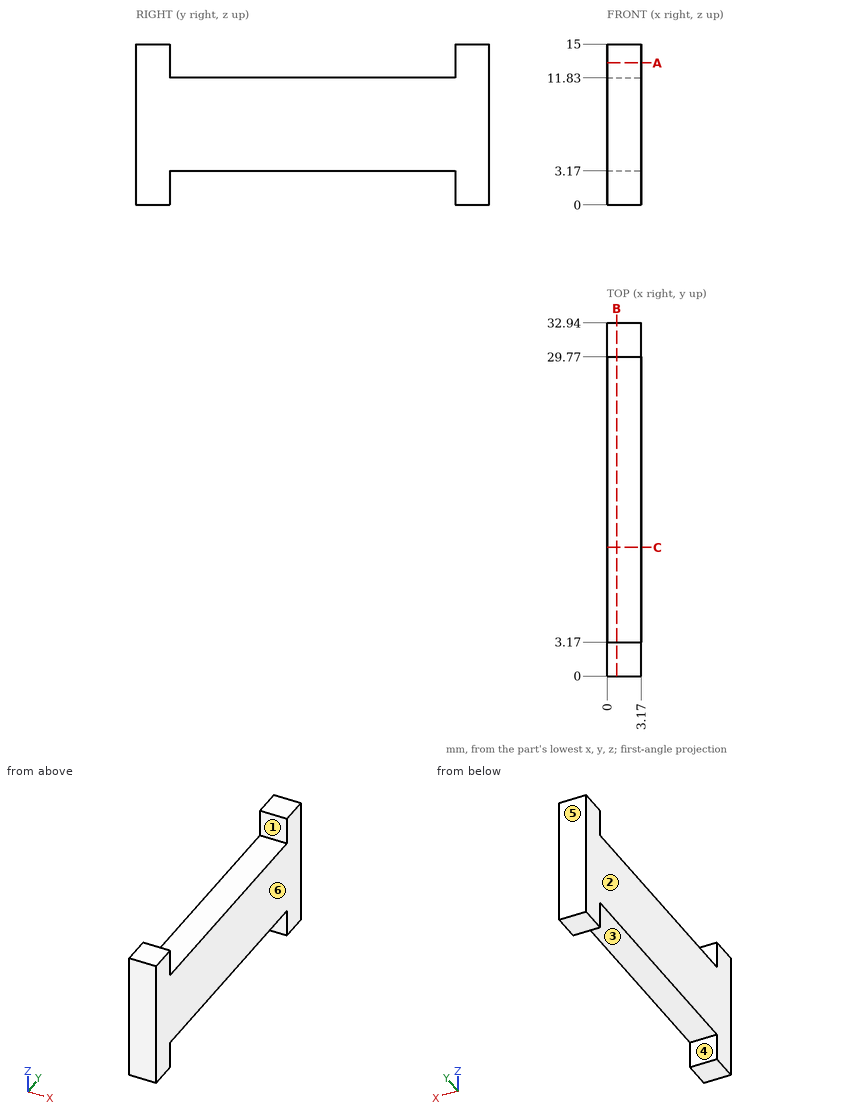
Geometry check sheet. Reference: drawing and pictorial views, mm from the part's lowest x, y, z. A direction names the side the tool comes from. Give positions to 0.01 mm unless a question says otherwise; leave off trailing zeros. Order: outer loops, then holes, each group sorted by start corner. A loop starts at its lowest first (then second) coordinate and runs counter-clockwise, first axis right, second up. Notation, with made-up numbers: M 3,-14 L 48,-14 A27 cw 48,7 Z; hole C 56,56 d9. An arc over 180 degrees is marked long. Return JSON: item names as keys, results as strings. Group by question number.
1) Mould release check, pull along Y, two halves, no side actions. Record for the marked faces 3, 4, 5 and 6: pulls with the +Y half, pulls with the -Y half, needs draft (parallel to the pull), parting line crosses it, or undercut.
2) Section check C-C on y = 12. Record the cut outline in (x, z).
3) Go/stop test with flat-tipped pins: pin 1 Ø1.6 at (x, y) = (1, 17.5) entering from -Z; pin 2 Ø1 at (x, y) = (2.5, 19.5) entering from +Z. Record where each tip stops, or that it passes through.
4) Section check A-A on z = 13.25. Record the cut outline in (x, y).
5) Section check B-B on x = 0.9. Record the cut outline in (y, z).
6) Scan lines: line 1 (Y direction, x = 1.3, z = 14.75); line 2 (Z direction, x = 1.9, y = 4). Record each from-to range of solid material in increasing order.
7) Access from +Z, -Z, +X, -X, +Y, -Y to the whole of each face (thin tool, end or side, straight path). Record for the marked faces 1 and 2.
Answer block:
{
 "1": {"face 3": "undercut", "face 4": "undercut", "face 5": "pulls with the +Y half", "face 6": "needs draft"},
 "2": {"outline": "M 0,3.17 L 3.17,3.17 L 3.17,11.83 L 0,11.83 Z"},
 "3": {"pin 1": "stops at z = 3.17", "pin 2": "stops at z = 11.83"},
 "4": {"outline": "M 0,0 L 3.17,0 L 3.17,3.17 L 0,3.17 Z; M 0,29.77 L 3.17,29.77 L 3.17,32.94 L 0,32.94 Z"},
 "5": {"outline": "M 0,0 L 3.17,0 L 3.17,3.17 L 29.77,3.17 L 29.77,0 L 32.94,0 L 32.94,15 L 29.77,15 L 29.77,11.83 L 3.17,11.83 L 3.17,15 L 0,15 Z"},
 "6": {"line 1": "y = 0 to 3.17, 29.77 to 32.94", "line 2": "z = 3.17 to 11.83"},
 "7": {"face 1": "+Z, +X, -X", "face 2": "+Z, -Z, -X, +Y, -Y"}
}
